Input: dimensioned drawing with shaded views. Units: mm. Origin: part minimum x, y, z. Coordinates: 2 decimals unless noted, no trailing zeros. Loops run counter-clockwise (first coordinate to the right, second up) from the corner with the lowest first, then second, coordinate; pieces in that order, holes last.
(1) Contact query for flat-ended pins moving along their axis: P1, Ø7.5, axis at y = 102.32, z = 7.32, coming from the +X side; P2, Ø4, axis at y = 137.68, z = 42.68, coming from the -X side. Output: stop coordinate, or through.
(2) Mould query, pull axis X, two halves, no side actions, for the marked faces 1, 2 and 3. Classes: released by +X, released by -X, zero draft, split by the parting line, or undercut.
(3) Section D-D, the plane x = 2. Return loops of the section in (y, z), then the cut area to 3 significant figures.
(4) Section C-C, the plane y = 137.68. Return loops of the section in (x, z).
(5) Line query: L1, parallel to Z at x = 4, y = 137.68; L2, parallel to Y at x = 2, z = 42.68; L3, parallel to Y at x = 6.6, z = 7.32. Output: solid intervals per line, ascending.
(6) Section B-B, the plane x = 8. Return loops of the section in (y, z).
(7) Section A-A, the plane z = 7.32. Return loops of the section in (x, y), then the cut area to 3 significant figures.
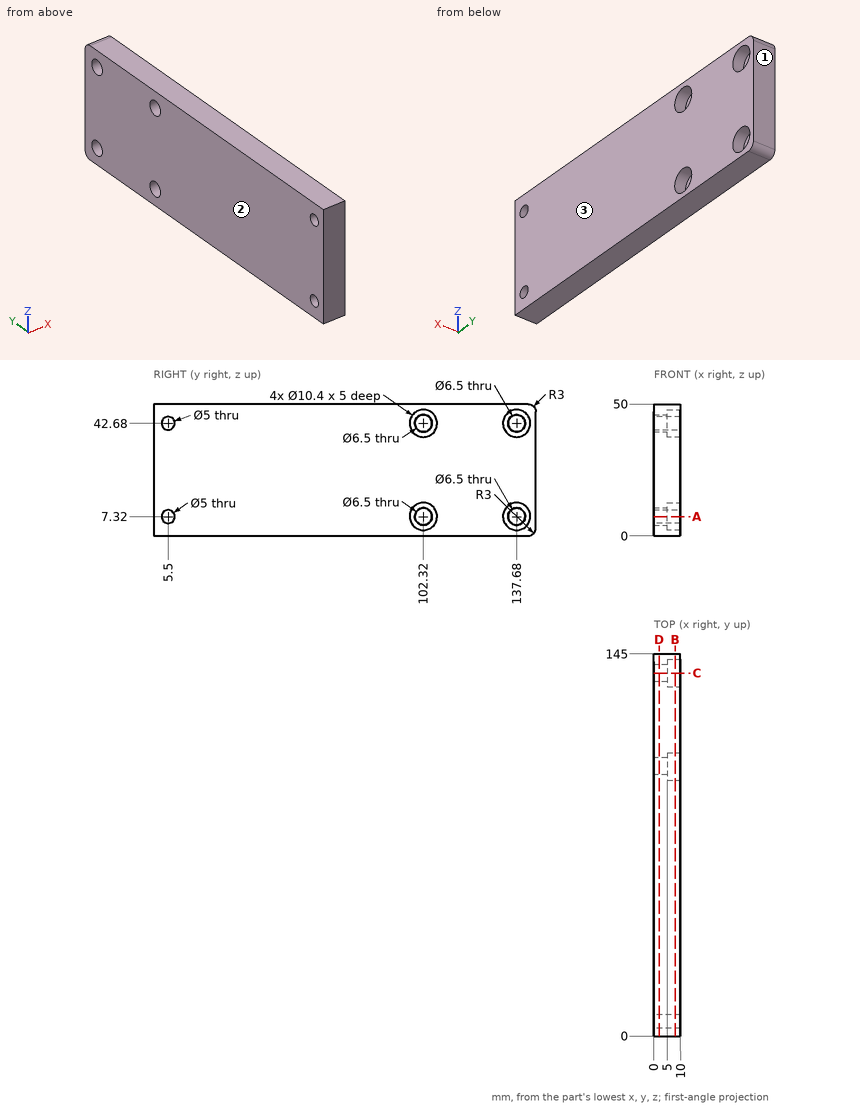
Report:
1. P1: stops at x = 5
1. P2: passes through
2. face 1: zero draft
2. face 2: released by -X
2. face 3: released by +X
3. outline: (0, 0) - (142, 0) arc R3 ccw to (145, 3) - (145, 47) arc R3 ccw to (142, 50) - (0, 50) - close; hole circle Ø5 at (5.5, 7.32); hole circle Ø5 at (5.5, 42.68); hole circle Ø6.5 at (102.32, 7.32); hole circle Ø6.5 at (102.32, 42.68); hole circle Ø6.5 at (137.68, 7.32); hole circle Ø6.5 at (137.68, 42.68)
3. area: 7,070 mm2
4. outline: (0, 0) - (10, 0) - (10, 2.12) - (5, 2.12) - (5, 4.07) - (0, 4.07) - close; (0, 10.57) - (5, 10.57) - (5, 12.52) - (10, 12.52) - (10, 37.48) - (5, 37.48) - (5, 39.43) - (0, 39.43) - close; (0, 45.93) - (5, 45.93) - (5, 47.88) - (10, 47.88) - (10, 50) - (0, 50) - close
5. L1: z = 0 to 4.07, 10.57 to 39.43, 45.93 to 50
5. L2: y = 0 to 3, 8 to 99.07, 105.57 to 134.43, 140.93 to 145
5. L3: y = 0 to 3, 8 to 97.12, 107.52 to 132.48, 142.88 to 145
6. outline: (0, 0) - (142, 0) arc R3 ccw to (145, 3) - (145, 47) arc R3 ccw to (142, 50) - (0, 50) - close; hole circle Ø5 at (5.5, 7.32); hole circle Ø5 at (5.5, 42.68); hole circle Ø10.4 at (102.32, 7.32); hole circle Ø10.4 at (102.32, 42.68); hole circle Ø10.4 at (137.68, 7.32); hole circle Ø10.4 at (137.68, 42.68)
7. outline: (0, 0) - (10, 0) - (10, 3) - (0, 3) - close; (0, 8) - (10, 8) - (10, 97.12) - (5, 97.12) - (5, 99.07) - (0, 99.07) - close; (0, 105.57) - (5, 105.57) - (5, 107.52) - (10, 107.52) - (10, 132.48) - (5, 132.48) - (5, 134.43) - (0, 134.43) - close; (0, 140.93) - (5, 140.93) - (5, 142.88) - (10, 142.88) - (10, 145) - (0, 145) - close
7. area: 1,230 mm2
